Check sheet for the modelled part. Datum: model origin and axes. Units: mm. Round coordinates to 2 decimals unless told otherwise and drop trailing zeros. Write each loop counter-clockwise with the first axis right and the second up, starting at its lowest first coordinate (ties: lowest second). Pieces come first, ordered by that corner, then holes. Notation, with made-up numbers: (40, -19) - (96, -19) arc R7 cw to (96, -9) - close; hole circle Ø4 at (-8, 65). An arc over 180 degrees is marked (long way). Answer as a JSON object with one key per item and string values. Group by question number.
Item 1: Thickness scan on line 1 (Y direction, x = 0, z = 0.75); line 2 (Y direction, x = -4, z = 0.7); line 3 (X direction, y = -60.5, z = 0.7). Record the ranges inside material, lowest first.
Item 2: Sectioned sample at C-C on z = 0.85. Record the boundary of the cut face in (x, y), plus the area to 3 significant figures.
Item 3: Sectioned sample at A-A on x = 0. Record the boundary of the cut face in (y, z).
Item 4: Release check for a two-part mould opening along Y. For faces 1 (the cylindrical face through (69.688, 71.216, 0.507)), 2 (the flat face through (62.7, -62.3, 0.5)), 3 (the flat face through (-62.7, 62.3, 0.5)), 4 (the flat face through (1, 1, 1)) record: pulls with the +Y half, pulls with the -Y half, needs draft (parallel to the pull), parting line crosses it, or undercut.
Item 5: Sectioned sample at B-B on y = 67. Record the boundary of the cut face in (x, z).
Item 6: Sectioned sample at D-D on x = -57. Record the boundary of the cut face in (y, z).
```python
from build123d import *

# Parameters (mm, degrees)
SKETCH1_R           = 6
BOSS_EXTRUDE1_DEPTH = 1
SKETCH2_R           = 5
CUT_EXTRUDE1_DEPTH  = 10


with BuildPart() as part:
    # Sketch1 → Boss-Extrude1 (new body)
    with BuildSketch(Plane.XY):
        Polygon((-75, 50), (-50, 75), (75, 75), (75, -50), (50, -75), (-50, -75), (-75, -50), align=None)
        with Locations((0, 50)):
            Circle(SKETCH1_R, mode=Mode.SUBTRACT)
    extrude(amount=BOSS_EXTRUDE1_DEPTH)

    # Sketch2 → Cut-Extrude1 (cut)
    with BuildSketch(Plane.XY.offset(1)):
        with Locations((67, 67)):
            Circle(SKETCH2_R)
    extrude(amount=-CUT_EXTRUDE1_DEPTH, mode=Mode.SUBTRACT)


solid = part.part
```
Completed:
{
 "1": {"line 1": "-75 to 44, 56 to 75", "line 2": "-75 to 45.53, 54.47 to 75", "line 3": "-64.5 to 64.5"},
 "2": {"outline": "(-75, -50) - (-50, -75) - (50, -75) - (75, -50) - (75, 75) - (-50, 75) - (-75, 50) - close; hole circle Ø12 at (0, 50); hole circle Ø10 at (67, 67)", "area": "21,400 mm²"},
 "3": {"outline": "(-75, 0) - (44, 0) - (44, 1) - (-75, 1) - close; (56, 0) - (75, 0) - (75, 1) - (56, 1) - close"},
 "4": {"face 1": "undercut", "face 2": "pulls with the -Y half", "face 3": "pulls with the +Y half", "face 4": "needs draft"},
 "5": {"outline": "(-58, 0) - (62, 0) - (62, 1) - (-58, 1) - close; (72, 0) - (75, 0) - (75, 1) - (72, 1) - close"},
 "6": {"outline": "(-68, 0) - (68, 0) - (68, 1) - (-68, 1) - close"}
}
